Design review of the part built by this model. Coordinates are the model's own, in mm. A direction names the side the tool comes from. Give positions to 0.01 mm unless a question says otherwise; leave off trailing zeros. Write each loop counter-clockwise with the first axis right and the second up, starting at its lowest first coordinate (ties: lowest second). Pieces come first, ordered by that corner, then holes. Notation, with made-up numbers: M 58.25,18.25 L 103.25,18.25 A21 cw 103.25,49.25 Z; hole C 84.25,-33 d5. An arc over 180 degrees is marked long. Use a Markdown table: item, result. Add a question column.
```python
from build123d import *

# Parameters (mm, degrees)
EXTRUDE_1_DEPTH = 3
M6X1_01_D       = 5
M6X1_01_DEPTH   = 9


with BuildPart() as part:
    # Эскиз1 → Повернуть1 (revolve)
    with BuildSketch(Plane.XY):
        with BuildLine():
            Line((0, 0), (0, 15))
            add(Edge.make_bspline(
                [(0, 15), (5.663028189, 9.794830304), (6, 0)],
                knots=[0, 0, 0, 1, 1, 1], degree=2))
            Line((6, 0), (0, 0))
        make_face()
    revolve(axis=Axis((0, 0, 0), (0, 1, 0)))

    # Эскиз2 → Бобышка-Вытянуть1 (add)
    with BuildSketch(Plane.XZ):
        Polygon((0, 6.92820323), (-6, 3.464101615), (-6, -3.464101615), (0, -6.92820323), (6, -3.464101615), (6, 3.464101615), align=None)
    extrude(amount=-EXTRUDE_1_DEPTH)

    # Отверстие обработанное метчиком M6x1.01
    with Locations(Plane(origin=(0, 0, 0), x_dir=(-1, 0, 0), z_dir=(0, -1, 0))):
        with Locations((0, 0)):
            Hole(M6X1_01_D / 2, depth=M6X1_01_DEPTH)


solid = part.part
```
(1) The part is to be moulded in two halves that separate along X. For faces 1 (the flat face through (0, 9, 0)), 2 (the flat face through (-1, 3, -6)), 3 (the flat face through (-3.042, 1.479, -5.172)), 4 (the flat face through (3.042, 1.479, 5.172)), say which applies: released by +X, released by -X, zero draft, split by the parting line, or undercut.
(2) For pin 1 (3 mm diameter, centred on y = 9, z = 0.5, fed in from -X); pin 2 (4 mm diameter, centred on x = 0, z = 0, fed in from -Y); pin 3 (1 mm diameter, centred on x = 3.5, y = 4.5, fed in from -Z); pin 4 (3 mm diameter, centred on y = 13, z = -5.5, fed in from +X), all flat-tipped, find the tip position at first contact; note any pin that passes through.
(3) Wall thickness on L1, parallel to Y at x = -0.75, z = 6; L2, parallel to Z at x = 0, y = 5.75; L3, parallel to Z at x = -1, y = 4: over which ranges is each line inside the solid? List them lowest first.
(4) Add section A-A on y = 1. Give the boundary of the cut face in (x, z).
(5) Machinability: for faces 5 (the flat face through (2.96, 1.48, -5.22)), 6 (the cylindrical face through (-0.54, 4.56, 2.44)), which of the approach directions +Z, -Z, +X, -X, +Y, -Y give a long, thin tool a straight path to every point of the face, cutting with its end or side? Answer none if there is none.
From the geometry:
| question | item | result |
|---|---|---|
| 1 | face 1 | undercut |
| 1 | face 2 | zero draft |
| 1 | face 3 | released by -X |
| 1 | face 4 | released by +X |
| 2 | pin 1 | stops at x = -4.74 |
| 2 | pin 2 | stops at y = 9 |
| 2 | pin 3 | stops at z = -4.65 |
| 2 | pin 4 | passes through |
| 3 | L1 | y = 0 to 3 |
| 3 | L2 | z = -5.25 to -2.5, 2.5 to 5.25 |
| 3 | L3 | z = -5.52 to -2.29, 2.29 to 5.52 |
| 4 | outline | M -6,-3.46 L 0,-6.93 L 6,-3.46 L 6,3.46 L 0,6.93 L -6,3.46 Z; hole C 0,0 d5 |
| 5 | face 5 | -Z, +X, +Y, -Y |
| 5 | face 6 | -Y |
